Build history of the part. All positions in model axes, mm. Face numbers are marked on the shaded views. A direction names the side the tool comes from. Round coordinates to 2 decimals unless told otherwise and drop trailing zeros. Order: outer loops, then holes, each group sorted by start corner. A loop starts at its lowest first (then second) coordinate and runs counter-clockwise, first axis right, second up. Notation, with made-up numbers: M 36,-37 L 51,-37 A21 cw 51,-18 Z; hole C -4,84 d11. An arc over 180 degrees is marked long. Use CSV: the item, a comma, the result in double quotes.
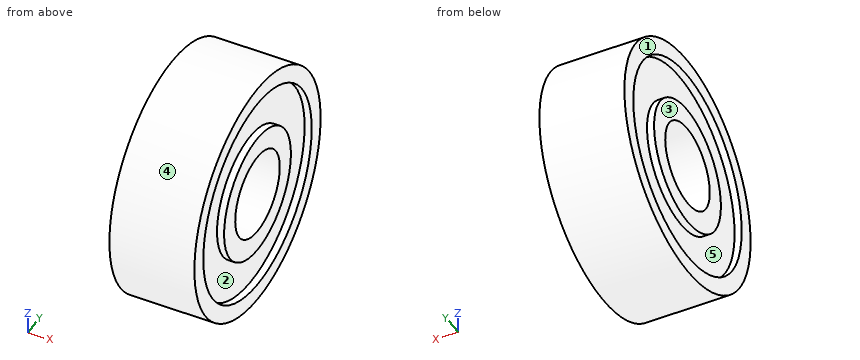
from build123d import *


with BuildPart() as part:
    # Croquis2 → Revolución1 (revolve)
    with BuildSketch(Plane.XY, mode=Mode.PRIVATE) as revoluci_n1_sk:
        Polygon((3, 7.3), (3, 8.5), (0, 8.5), (0, 3), (3, 3), (3, 4.5), (2.5, 4.5), (2.5, 7.3), align=None)
        Polygon((0, 3), (0, 8.5), (-3, 8.5), (-3, 7.3), (-2.5, 7.3), (-2.5, 4.5), (-3, 4.5), (-3, 3), align=None)
    revolve(revoluci_n1_sk.sketch.rotate(Axis((6.771887169, 0, 0), (-1, 0, 0)), 90), axis=Axis((6.771887169, 0, 0), (-1, 0, 0)))


solid = part.part
(1) Two-plate mould, pull along Z, no slides. Class the marked faces 3, 4 and 5: released by +Z, released by -Z, zero draft, split by the parting line, or undercut.
Answer block:
face 3,"zero draft"
face 4,"split by the parting line"
face 5,"undercut"
(2) Drop flat-ended pins along their axis: pin 1 (9 mm diameter, centred on y = 0, z = 0, fed in from -X); pin 2 (1.5 mm diameter, centred on x = -0.5, z = -5, fed in from -Y); pin 3 (2 mm diameter, centred on x = -0.5, y = -4, fed in from +Z); pin 4 (3 mm diameter, centred on x = -2, z = -5.5, fed in from +Y). Give the stop position or say it passes through.
Answer block:
pin 1,"stops at x = -3"
pin 2,"stops at y = -7.36"
pin 3,"stops at z = 7.95"
pin 4,"stops at y = 7.5"
(3) Tool access for the marked faces 1 and 2: list every direction of +Z, -Z, +X, -X, +Y, -Y with a clear straight run to the whole face (end or side of a thin tool).
Answer block:
face 1,"+Z, -Z, -X, +Y, -Y"
face 2,"+X"
(4) Cut at C-C, the plane x = 1.3. Give the cut face in (y, z).
Answer block:
outline,"C 0,0 d17; hole C 0,0 d6"
(5) Cut at D-D, the plane y = -6.25. Give the cut face in (x, z), and give its area (3 significant figures).
Answer block:
outline,"M -3,-5.76 L 3,-5.76 L 3,-3.77 L 2.5,-3.77 L 2.5,3.77 L 3,3.77 L 3,5.76 L -3,5.76 L -3,3.77 L -2.5,3.77 L -2.5,-3.77 L -3,-3.77 Z"
area,"61.6 mm²"
(6) Cut at A-A, the plane y = 0. Give the cut face in (x, z).
Answer block:
outline,"M -3,-8.5 L 3,-8.5 L 3,-7.3 L 2.5,-7.3 L 2.5,-4.5 L 3,-4.5 L 3,-3 L -3,-3 L -3,-4.5 L -2.5,-4.5 L -2.5,-7.3 L -3,-7.3 Z; M -3,3 L 3,3 L 3,4.5 L 2.5,4.5 L 2.5,7.3 L 3,7.3 L 3,8.5 L -3,8.5 L -3,7.3 L -2.5,7.3 L -2.5,4.5 L -3,4.5 Z"
(7) Wall check: line 1 (Y direction, x = 2.7, z = 0); line 2 (Y direction, x = -0.05, z = 0); line 3 (X direction, y = 4.5, z = -2.75). Give the ranges that are in metal, low to high. Write a range as from..to.
Answer block:
line 1,"y = -8.5..-7.3, -4.5..-3, 3..4.5, 7.3..8.5"
line 2,"y = -8.5..-3, 3..8.5"
line 3,"x = -2.5..2.5"
